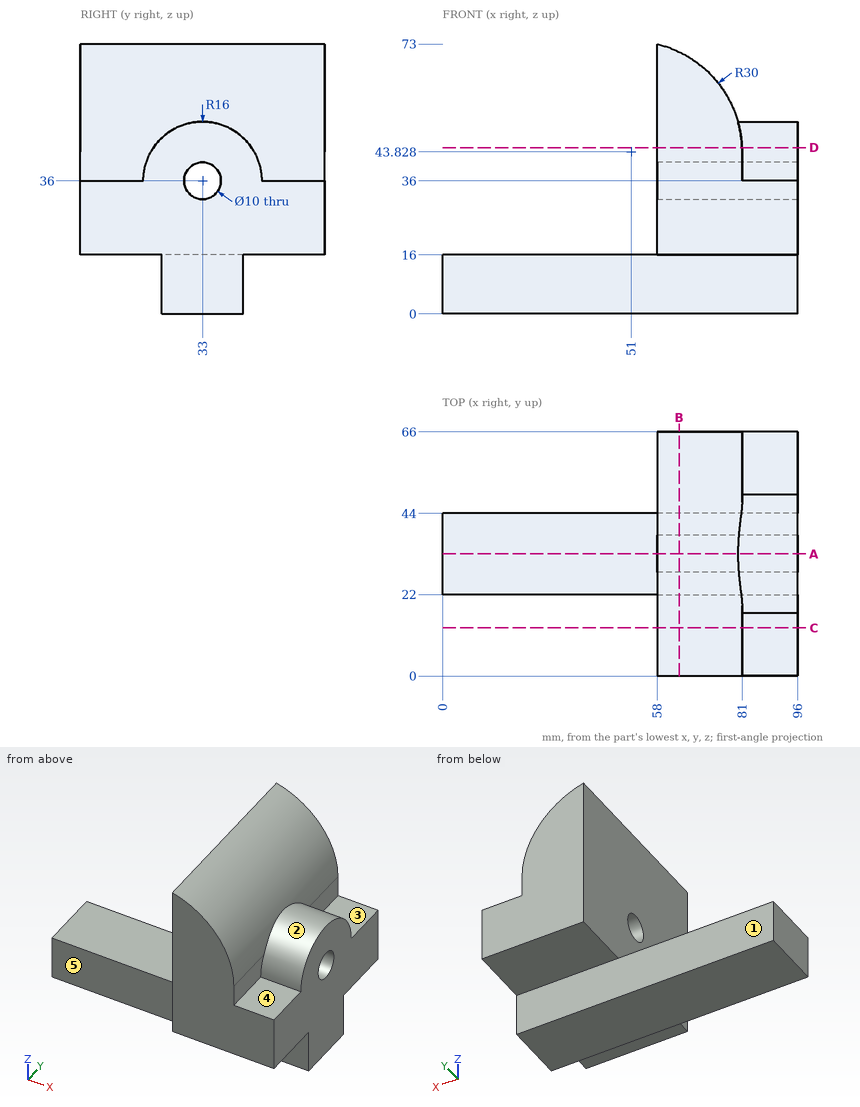
Part print with two shaded views. Sizes in mm from the minimum x, y, z corner. A direction names the side the tool comes from. Round coordinates to 2 decimals unless told otherwise and drop trailing zeros. Loops run counter-clockwise (first coordinate to the right, second up) from the corner with the lowest first, then second, coordinate; pieces in that order, holes last. Notation, with made-up numbers: (54.25, 29) - (87.25, 29) arc R18 cw to (87.25, 34) - close; hole circle Ø7 at (75, -13.75). An arc over 180 degrees is marked (long way). Answer as a JSON object with one key per item and string values.
Item 1: Band-saw the part on D-D on z = 45. List the corners of the cut face in (x, y), plus the area to 3 significant figures.
Output:
{"outline": "(58, 0) - (80.98, 0) - (80.98, 19.77) - (96, 19.77) - (96, 46.23) - (80.98, 46.23) - (80.98, 66) - (58, 66) - close", "area": "1,910 mm2"}
Item 2: Tool access for the marked faces 1, 2, 3, 4 and 5: list every direction of +Z, -Z, +X, -X, +Y, -Y with a clear straight run to the whole face (end or side of a thin tool).
Output:
{"face 1": "-Z, +X, -X, +Y", "face 2": "+Z, +X", "face 3": "+Z, +X, +Y", "face 4": "+Z, +X, -Y", "face 5": "-Z, +X, -X, -Y"}
Item 3: Band-saw the part on A-A on y = 33. List the corners of the cut face in (x, z), plus the area to 3 significant figures.
Output:
{"outline": "(0, 0) - (96, 0) - (96, 31) - (58, 31) - (58, 16) - (0, 16) - close; (58, 41) - (96, 41) - (96, 52) - (79.87, 52) arc R30 ccw to (58, 73) - close", "area": "2,840 mm2"}
Item 4: Wall check: L1, parallel to Y at x = 72.5, z = 36; L2, parallel to Y at x = 59, z = 7.5; L3, parallel to Y at x = 70.5, z = 37. Give the ranges that are in metal, low to high.
Output:
{"L1": "0 to 28, 38 to 66", "L2": "22 to 44", "L3": "0 to 28.1, 37.9 to 66"}
Item 5: Pin check, flat tips, straight feed: pin 1 (17.5 mm diameter, centred on x = 52, z = 9.5, fed in from -Y); pin 2 (10 mm diameter, centred on x = 27, z = 20, fed in from +Y); pin 3 (2.5 mm diameter, centred on y = 7.5, z = 39, fed in from +X); pin 4 (1.5 mm diameter, centred on y = 23, z = 15, fed in from -X). Stop position of each tip, or through.
Output:
{"pin 1": "y = 22", "pin 2": "y = 44", "pin 3": "x = 81", "pin 4": "x = 0"}
Item 6: Band-saw the part on C-C on y = 13. List the corners of the cut face in (x, z), plus the area to 3 significant figures.
Output:
{"outline": "(58, 16) - (96, 16) - (96, 36) - (81, 36) - (81, 43.83) arc R30 ccw to (58, 73) - close", "area": "1,440 mm2"}
Item 7: Band-saw the part on B-B on x = 64. List the corners of the cut face in (y, z) (3 decimals), plus the area to 3 significant figures.
Output:
{"outline": "(0, 16) - (22, 16) - (22, 0) - (44, 0) - (44, 16) - (66, 16) - (66, 70.865) - (0, 70.865) - close; hole circle Ø10 at (33, 36)", "area": "3,890 mm2"}
